from build123d import *

# Parameters (mm, degrees)
F0_R     = 11
F1_DEPTH = 15
F2_R     = 4.5
F3_DEPTH = 2
F4_R     = 1.6
F5_DEPTH = 5


with BuildPart() as f1:
    # F0 (on Front) → F1 (new body)
    with BuildSketch(Plane.XZ):
        Circle(F0_R)
    extrude(amount=F1_DEPTH)

    # F2 (on face) → F3 (join)
    with BuildSketch(Plane(origin=(0, 0, 0), x_dir=(-1, 0, 0), z_dir=(0, 1, 0))):
        Circle(F2_R)
    extrude(amount=F3_DEPTH)

    # F4 (on face) → F5 (cut)
    with BuildSketch(Plane(origin=(0, 2, 0), x_dir=(-1, 0, 0), z_dir=(0, 1, 0))):
        Circle(F4_R)
    extrude(amount=-F5_DEPTH, mode=Mode.SUBTRACT)


solid = f1.part
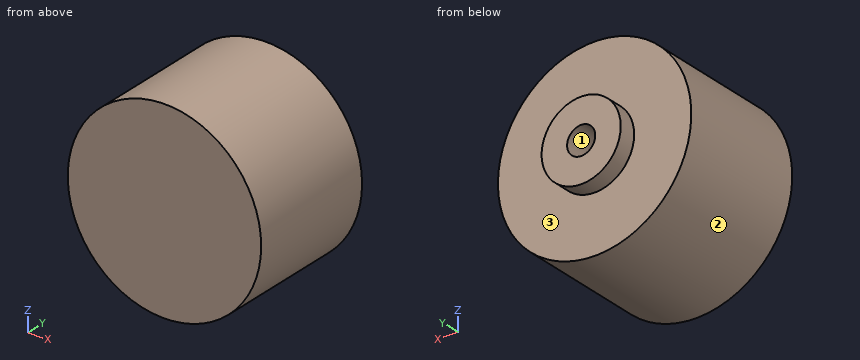
The listing builds one solid part. Answer for the finished solid, in the listing's coordinates (mm). Face numbers are marked on the shaded views. Round coordinates to 2 decimals unless told otherwise and drop trailing zeros. Write each loop counter-clockwise with the first axis right and the second up, starting at its lowest first coordinate (ties: lowest second). Pieces come first, ordered by that corner, then holes. Notation, with made-up numbers: M -10.75,-35 L -4.75,-35 A6 cw -4.75,-24 Z; hole C -4,-34.5 d2. An arc over 180 degrees is marked long. Write each question's results on one line, items separated by ' | '. Start each with the question number.
Item 1: The mould has two halves that part along Z. Classify the marked faces 1, 2 and 3: +Z half, -Z half, draft (parallel to the pull), parting line (faces both ways), or undercut.
Item 2: Find section B-B on x = 0. Write down the section's boundary in (y, z).
Item 3: Find section A-A on y = 0.5. Write down the section's boundary in (x, z).
Item 4: Given pin 1 Ø3 at (y, z) = (-2.5, 7.5) entering from -X; pin 2 Ø2 at (y, z) = (-9, -5.5) entering from +X; pin 3 Ø2 at (x, y) = (3, -11.5) entering from -Z, each flat-ended and moving along its own axis, determine where each tip first touches the part or whether it passes through.
Item 5: Straight lines are drawn through the part: probe 1 along Z at (x, y) = (0, -1.5); probe 2 along Z at (x, y) = (0, 0.6); probe 3 along Y at (x, z) = (6.75, 6.5). For each, find the intervals that lie inside material, in ascending order.
Item 6: Find section C-C on z = 0. Write down the section's boundary in (x, y), and give its area (3 significant figures).
Item 7: Find section D-D on y = -5.25. Write down the section's boundary in (x, z), and give its area (3 significant figures).
Answer block:
1) face 1: undercut | face 2: parting line | face 3: draft
2) outline: M -15,-11 L 0,-11 L 0,-4.5 L 2,-4.5 L 2,-1.6 L -3,-1.6 L -3,1.6 L 2,1.6 L 2,4.5 L 0,4.5 L 0,11 L -15,11 Z
3) outline: C 0,0 d9; hole C 0,0 d3.2
4) pin 1: stops at x = -9.22 | pin 2: stops at x = 10.04 | pin 3: stops at z = -10.82
5) probe 1: z = -11 to -1.6, 1.6 to 11 | probe 2: z = -4.5 to -1.6, 1.6 to 4.5 | probe 3: y = -15 to 0
6) outline: M -11,-15 L 11,-15 L 11,0 L 4.5,0 L 4.5,2 L 1.6,2 L 1.6,-3 L -1.6,-3 L -1.6,2 L -4.5,2 L -4.5,0 L -11,0 Z | area: 332 mm²
7) outline: C 0,0 d22 | area: 380 mm²
